Source: three-view drawing plus pictorial views. Frame: mm from the lowest corner of the part. A direction names the side the tool comes from. Round coordinates to 2 decimals unless told otherwise and drop trailing zeros. Order: outer loops, then holes, each group sorted by start corner. A loop starts at its lowest first (then second) coordinate and runs counter-clockwise, first axis right, second up. Notation, with made-up numbers: (30, 35.5) - (54, 35.5) arc R24 ccw to (54, 67.5) - close; hole circle Ø6 at (2, 22.25). An arc over 180 degrees is marked (long way). Use one line per item in the form item = value. Start each with the question number.
Q1. Set-up query: the marked faces 1 and 2. Return all of +Z, -Z, +X, -X, +Y, -Y with unobstructed straight access to the full face (end or side cutting, diameter ignored); none if empty.
Q2. Ray query, line 1 (X direction, y = 24.16, z = 8); line 2 (Z direction, x = 11, y = 30.5); line 3 (X direction, y = 15, z = 2.25). Return the intervals inside material, ascending. Write a range as [from, to].
Q3. Draft query along Y for the marked faces 3, 4 and 5. Return one class per face: released by +Y, released by -Y, zero draft, split by the parting line, or undercut.
Q4. Pin query (flat end, axial travel): pin 1 Ø5 at (x, y) = (11.5, 35.5) entering from -Z; pin 2 Ø1.2 at (y, z) = (26, 2.5) entering from -X; pin 3 Ø0.7 at (x, y) = (12, 24.16) entering from -Z. Return the tip coordinate at first contact, or that it passes through.
Q5. Cut plane C-C, the plane x = 7.75. Return the cut outline in (y, z).
Q6. Cut plane A-A, the plane y = 29.24. Return the cut outline in (x, z), and give its area (3 significant figures).
Q7. Cut plane B-B, the plane z = 2.75. Return the cut outline in (x, y).
Q8. Cut plane D-D, the plane z = 7.5. Give the number of separate pieces and of enclosed holes in the cut face, and give its area (3 significant figures).
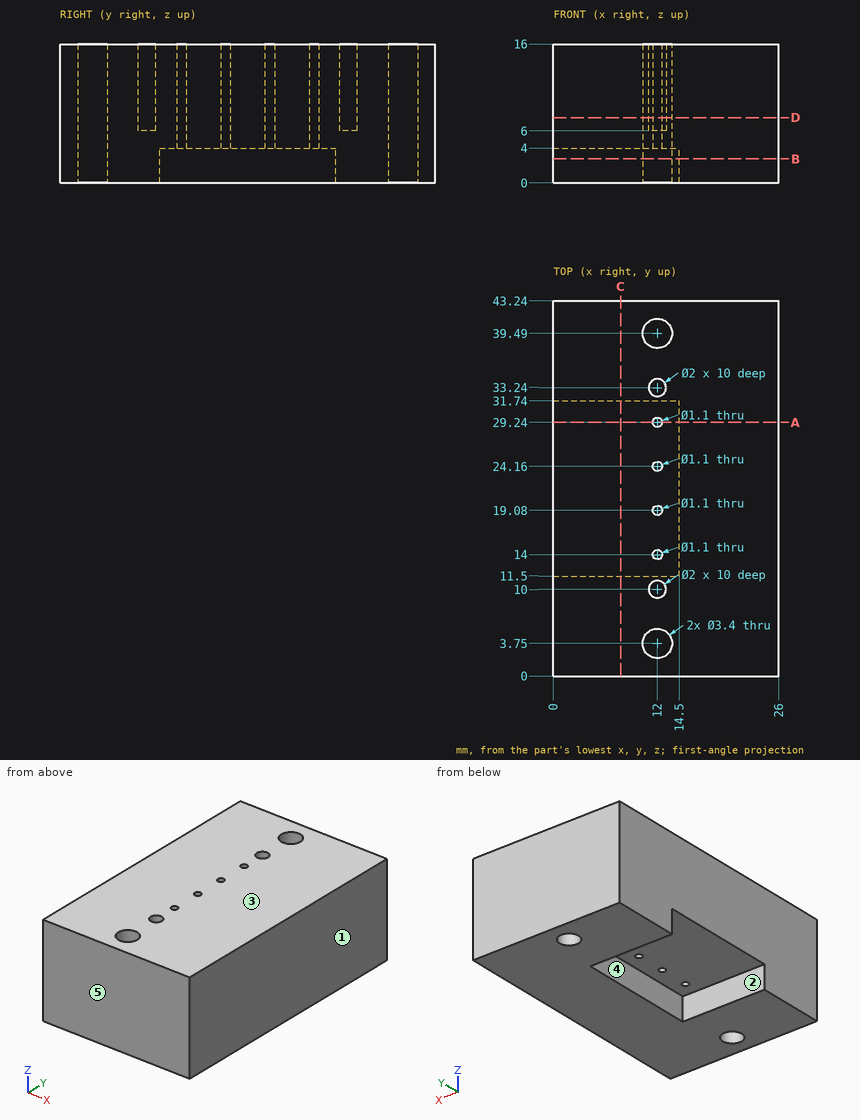
Completed:
q1.face_1 = +Z, -Z, +X, +Y, -Y
q1.face_2 = -Z, -X
q2.line_1 = [0, 11.45], [12.55, 26]
q2.line_2 = [4, 16]
q2.line_3 = [14.5, 26]
q3.face_3 = zero draft
q3.face_4 = undercut
q3.face_5 = released by -Y
q4.pin_1 = 0
q4.pin_2 = 14.5
q4.pin_3 = through
q5.outline = (0, 0) - (11.5, 0) - (11.5, 4) - (31.74, 4) - (31.74, 0) - (43.24, 0) - (43.24, 16) - (0, 16) - close
q6.outline = (0, 4) - (11.45, 4) - (11.45, 16) - (0, 16) - close; (12.55, 4) - (14.5, 4) - (14.5, 0) - (26, 0) - (26, 16) - (12.55, 16) - close
q6.area = 345 mm2
q7.outline = (0, 0) - (26, 0) - (26, 43.24) - (0, 43.24) - (0, 31.74) - (14.5, 31.74) - (14.5, 11.5) - (0, 11.5) - close; hole circle Ø3.4 at (12, 3.75); hole circle Ø3.4 at (12, 39.49)
q8.separate_pieces = 1
q8.enclosed_holes = 8
q8.area = 1,100 mm2
